from build123d import *

# Parameters (mm, degrees)
F0_W     = 565.15
F0_H     = 412.75
F1_DEPTH = 18
F2_R     = 159.940625
F3_DEPTH = 18.001
F5_D     = 3.175
F5_DEPTH = 3.175
F5_TIP   = 0.9538662327


with BuildPart() as f1:
    # F0 (on Top) → F1 (new body)
    with BuildSketch(Plane.XY):
        Rectangle(F0_W, F0_H)
    extrude(amount=F1_DEPTH)

    # F2 (on face) → F3 (cut, through all)
    with BuildSketch(Plane.XY.offset(18)):
        Circle(F2_R)
    extrude(amount=-F3_DEPTH, mode=Mode.SUBTRACT)

    # F5
    with Locations(Plane(origin=(0, 0, 0), x_dir=(1, 0, 0), z_dir=(0, 0, -1))):
        with Locations((-257.175, -180.975), (-212.725, -180.975), (-212.725, -144.4625), (-257.175, -144.4625), (-257.175, -107.95), (-212.725, -107.95), (-257.175, 107.95), (-212.725, 107.95), (-257.175, 144.4625), (-212.725, 144.4625), (-257.175, 180.975), (-212.725, 180.975), (212.725, 180.975), (257.175, 180.975), (257.175, 144.4625), (212.725, 144.4625), (212.725, 107.95), (257.175, 107.95), (212.725, -107.95), (257.175, -107.95), (212.725, -144.4625), (257.175, -180.975), (257.175, -144.4625), (212.725, -180.975)):
            Hole(F5_D / 2, depth=F5_DEPTH)
            with Locations((0, 0, -(F5_DEPTH + F5_TIP / 2))):  # 118° drill point
                Cone(0, F5_D / 2, F5_TIP, mode=Mode.SUBTRACT)


solid = f1.part
The listing builds one solid part. Answer for the finished solid, in the listing's coordinates (mm). Coordinates: 2 decimals unless noted, no trailing zeros. Write each loop counter-clockwise with the first axis right and the second up, starting at its lowest first coordinate (ties: lowest second). Pieces come first, ordered by that corner, then holes. Notation, with made-up numbers: M -11.5,87 L 31.5,87 A16 cw 31.5,108 Z; hole C -29,-37 d3. An arc over 180 degrees is marked long. Write each question's results on one line, items separated by ' | '.
Item 1: For a pull along Y with two mould halves and no side action, classify faces 1 (the face through (-130, 95, 18)), 2 (the face through (-4, 206.375, 9)), 3 (the face through (152.555, 48.042, 9.126)), 4 (the face through (-4, -206.375, 9)) as released by +Y, released by -Y, zero draft, split by the parting line, or undercut.
Answer below:
face 1: zero draft | face 2: released by +Y | face 3: undercut | face 4: released by -Y
Item 2: The part is cut by section C-C on z = 10.5. Determine the outline of the cut face in (x, y) (3 decimals), and give its area (3 significant figures).
Answer below:
outline: M -282.575,-206.375 L 282.575,-206.375 L 282.575,206.375 L -282.575,206.375 Z; hole C 0,0 d319.881 | area: 153,000 mm2
Item 3: The part is cut by section B-B on x = 0. Determine the outline of the cut face in (y, z) (3 decimals).
Answer below:
outline: M -206.375,0 L -159.941,0 L -159.941,18 L -206.375,18 Z; M 159.941,0 L 206.375,0 L 206.375,18 L 159.941,18 Z
Item 4: Consider probe 1 along Y at (x, z) = (0, 10.5) (3 decimals); probe 2 along X at (y, z) = (5.5, 12) (3 decimals); probe 3 along Y at (x, z) = (65, 9) (3 decimals). Determine where each line is inside the solid, lowest interval first. Write a range as [from, to].
Answer below:
probe 1: [-206.375, -159.941], [159.941, 206.375] | probe 2: [-282.575, -159.846], [159.846, 282.575] | probe 3: [-206.375, -146.137], [146.137, 206.375]
Item 5: Given P1, Ø2.5, axis at x = 212.725, y = -180.975, coming from the -Z side; P2, Ø3, axis at x = -212.725, y = 180.975, coming from the -Z side; P3, Ø1.9, axis at x = 212.725, y = 107.95, coming from the -Z side, each flat-ended and moving along its own axis, determine where each tip first touches the part or whether it passes through.
Answer below:
P1: z = 3.38 | P2: z = 3.23 | P3: z = 3.56
Item 6: The part is cut by section A-A on y = 0. Determine the outline of the cut face in (x, z) (3 decimals), and give its area (3 significant figures).
Answer below:
outline: M -282.575,0 L -159.941,0 L -159.941,18 L -282.575,18 Z; M 159.941,0 L 282.575,0 L 282.575,18 L 159.941,18 Z | area: 4,410 mm2
